Autodesk Inventor part; units mm, degrees
ref_plane "YZ Plane" through (0, 0, 0) normal (1, 0, 0) x (0, 1, 0)
ref_plane "XZ Plane" through (0, 0, 0) normal (0, 1, 0) x (-1, 0, 0)
ref_plane "XY Plane" through (0, 0, 0) normal (0, 0, 1) x (1, 0, 0)
sketch "스케치1" plane through (0, 0, 0) normal (0, 1, 0) x (-1, 0, 0)
  circle A0 centre (0, 0) radius 15
  circle A1 centre (0, 0) radius 17.5
  dimension "d0" = 30
  dimension "d1" = 35
extrude "돌출1" add sketch "스케치1" along normal blind 2
sketch "스케치2" plane through (0, 2, 0) normal (0, 1, 0) x (1, 0, 0)
  line L0 (0, 0) -> (-15, 0)
  circle A0 centre (0, 0) radius 15
  line L1 (0, 0) -> (-14.0954, -5.1303)
  line L2 (0, 0) -> (15, 0) construction
  line L3 (0, 0) -> (-14.0954, 5.1303)
  line L4 (0, 0) -> (11.4907, 9.6418)
  line L5 (0, 0) -> (2.6047, 14.7721)
  line L6 (0, 0) -> (12.8233, -7.7822)
  line L7 (0, 0) -> (4.8209, -14.2042)
  arc A1 (-14.0954, 5.1303) -> (-14.0954, -5.1303) centre (0, 0) ccw
  arc A2 (4.8209, -14.2042) -> (12.8233, -7.7822) centre (0, 0) ccw
  arc A3 (11.4907, 9.6418) -> (2.6047, 14.7721) centre (0, 0) ccw
  circle A4 centre (0, 0) radius 5
  point P0 (-7.5, 0)
  point P1 (0.8682, 4.924)
  point P2 (3.8302, 3.2139)
  point P3 (4.2744, -2.5941)
  point P4 (1.607, -4.7347)
  point P5 (-4.6985, 1.7101)
  point P6 (-4.6985, -1.7101)
  dimension "d15" = 10
extrude "돌출2" add sketch "스케치2" against normal blind 2 contours A4 L1 A0 L0 | L0 A0 L3 A4 | A4 L5 A0 L4 | L6 A0 L7 A4
sketch "스케치3" plane through (0, 2, 0) normal (0, 1, 0) x (1, 0, 0)
  circle A0 centre (0, 0) radius 15
  circle A1 centre (0, 0) radius 17.5
  dimension "d18" = 30
extrude "돌출3" add sketch "스케치3" along normal blind 2
properties part number "fan_num5_1"
Read the model definition and answer for the solid it produces. Units are mm, in the model's axes. A direction names the side the tool comes from. Give positions to 0.01 mm unless a question says otherwise; leave off trailing zeros. Write each loop counter-clockwise with the first axis right and the second up, starting at its lowest first coordinate (ties: lowest second). Pieces come first, ordered by that corner, then holes. Notation, with made-up numbers: (52, -18.5) -> (109, -18.5) arc R10 cw to (109, -5.5) -> close; hole circle Ø7 at (27.5, -19.5). An arc over 180 degrees is marked (long way). Answer as a JSON object with one key per item and string values. Group by question number.
1) Find section B-B (z = 0). Write down the section's boundary in (x, y).
2) The mould has two halves that part along Z. Classify faces 4 (the flat face through (13, 4, -8)), 5 (the flat face through (6, 2, 8)), 6 (the flat face through (5, 2, -9)): +Z half, -Z half, draft (parallel to the pull), parting line (faces both ways), or undercut.
3) Each of these flat-tipped pins is pushed along its axis until it touches: P1, Ø1.5, axis at x = 1, y = 1.5, coming from the +Z side; P2, Ø1.5, axis at x = -0.5, z = -12, coming from the +Y side; P3, Ø3, axis at x = 4, z = -9, coming from the +Y side; P4, Ø1.5, axis at y = 1, z = 2.5, coming from the -X side. Where does it stop, or does it pass through?
4) Find section C-C (x = -12.5). Write down the section's boundary in (y, z).
5) Consider L1, parallel to Z at x = 0, y = 2.5; L2, parallel to Z at x = -13, y = 1.1. Determine where each line is inside the solid, lowest interval first. Write a range as from..to.
6) A tool of negligible diameter and unlimited length cuts with its end or side. For faces 1 (the cylindrical face through (3, 1, -4)), 2 (the flat face through (-11, 2, 0)), 3 (the flat face through (4, 0, -4)), from which of +Z, -Z, +X, -X, +Y, -Y can it reach the whole face along a straight path? Write none if from no direction.
7) Find section A-A (x = 0). Write down the section's boundary in (y, z).
8) Find section D-D (z = -7). Write down the section's boundary in (x, y).
Values follow:
{
 "1": {"outline": "(-17.5, 0) -> (-5, 0) -> (-5, 2) -> (-15, 2) -> (-15, 4) -> (-17.5, 4) -> close; (15, 0) -> (17.5, 0) -> (17.5, 4) -> (15, 4) -> close"},
 "2": {"face 4": "draft", "face 5": "undercut", "face 6": "undercut"},
 "3": {"P1": "stops at z = 17.5", "P2": "passes through", "P3": "stops at y = 2", "P4": "stops at x = -17.41"},
 "4": {"outline": "(0, -12.25) -> (4, -12.25) -> (4, -8.29) -> (0, -8.29) -> close; (0, -4.55) -> (2, -4.55) -> (2, 4.55) -> (0, 4.55) -> close; (0, 8.29) -> (4, 8.29) -> (4, 12.25) -> (0, 12.25) -> close"},
 "5": {"L1": "z = -17.5..-15, 15..17.5", "L2": "z = -11.72..-7.48, -4.73..4.73, 7.48..11.72"},
 "6": {"face 1": "+Y, -Y", "face 2": "+Y", "face 3": "+Z, -Z, +X, -X, -Y"},
 "7": {"outline": "(0, -17.5) -> (4, -17.5) -> (4, -15) -> (0, -15) -> close; (0, 15) -> (4, 15) -> (4, 17.5) -> (0, 17.5) -> close"},
 "8": {"outline": "(-16.04, 0) -> (-13.27, 0) -> (-13.27, 4) -> (-16.04, 4) -> close; (1.23, 0) -> (8.34, 0) -> (8.34, 2) -> (1.23, 2) -> close; (13.27, 0) -> (16.04, 0) -> (16.04, 4) -> (13.27, 4) -> close"}
}
